Model file for the job. Use its own axes, mm. Face numbers are marked on the shaded views. A direction names the side the tool comes from. Coordinates: 2 decimals unless noted, no trailing zeros. Write each loop counter-clockwise with the first axis right and the second up, starting at its lowest first coordinate (ties: lowest second). Pieces come first, ordered by that corner, then holes.
Q1. Band-saw the part on A-A, the plane x = 0. Write the cut outline in (y, z).
Q2. Band-saw the part on D-D, the plane y = -14. Write the cut outline in (x, z), plus the area to 3 significant figures.
Q3. Band-saw the part on C-C, the plane z = 4. Write the cut outline in (x, y), plus the area to 3 significant figures.
Q4. Pin check, flat tips, straight feed: P1, Ø5, axis at x = -19.5, y = -17.5, coming from the -Z side; P2, Ø4, axis at y = 14, z = -3.5, coming from the +X side; P3, Ø4, axis at x = -10.5, z = -4, coming from the +Y side. Stop position of each tip, or through.
Q5. Drill centre lines: probe 1 along Y at (x, z) = (0, 0.5); probe 2 along X at (y, z) = (-2, -1.5); probe 3 along Z at (x, y) = (9.5, 22). Where is each one in solid material? Low to high.
Q6. Which spindle directions (+Z, -Z, +X, -X, +Y, -Y) get a long thin tool onto all of the face, cutting with end or side? Do the marked faces 1 and 2. Say none if no direction does.
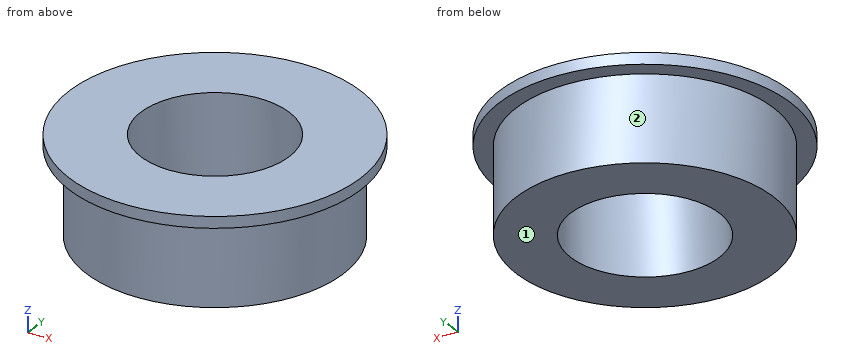
from build123d import *

# Parameters (mm, degrees)
SKETCH_R     = 22.5
PAD_DEPTH    = 7.5
SKETCH001_R  = 25.5
PAD001_DEPTH = 2
SKETCH002_R  = 13
POCKET_DEPTH = 44.501


with BuildPart() as part:
    # Sketch → Pad (new body, symmetric)
    with BuildSketch(Plane.XY):
        Circle(SKETCH_R)
    extrude(amount=PAD_DEPTH, both=True)

    # Sketch001 (on Face3 of Pad) → Pad001 (join)
    with BuildSketch(Plane.XY.offset(7.5)):
        Circle(SKETCH001_R)
    extrude(amount=PAD001_DEPTH)

    # Sketch002 → Pocket (cut, through all)
    with BuildSketch(Plane.XY.offset(37)):
        Circle(SKETCH002_R)
    extrude(amount=-POCKET_DEPTH, mode=Mode.SUBTRACT)


solid = part.part
Answer sheet:
1. outline: (-25.5, 7.5) - (-22.5, 7.5) - (-22.5, -7.5) - (-13, -7.5) - (-13, 9.5) - (-25.5, 9.5) - close; (13, -7.5) - (22.5, -7.5) - (22.5, 7.5) - (25.5, 7.5) - (25.5, 9.5) - (13, 9.5) - close
2. outline: (-21.31, 7.5) - (-17.61, 7.5) - (-17.61, -7.5) - (17.61, -7.5) - (17.61, 7.5) - (21.31, 7.5) - (21.31, 9.5) - (-21.31, 9.5) - close
2. area: 614 mm2
3. outline: circle Ø45 at (0, 0); hole circle Ø26 at (0, 0)
3. area: 1,060 mm2
4. P1: stops at z = 7.5
4. P2: stops at x = 19.03
4. P3: stops at y = 20.83
5. probe 1: y = -22.5 to -13, 13 to 22.5
5. probe 2: x = -22.41 to -12.85, 12.85 to 22.41
5. probe 3: z = 7.5 to 9.5
6. face 1: -Z, +X, -X, +Y, -Y
6. face 2: -Z
